Source: CAD feature listing. Evaluate the final solid. Frame: model axes, mm. Face numbers are marked on the shaded views. A direction names the side the tool comes from. Coordinates: 2 decimals unless noted, no trailing zeros. Order: outer loops, then holes, each group sorted by start corner. A loop starts at its lowest first (then second) coordinate and runs counter-clockwise, first axis right, second up.
```python
from build123d import *

# Parameters (mm, degrees)
BASE_FLANGE1_DEPTH           = 3.175
SKETCH7_R                    = 3.15
CUT_EXTRUDE3_DEPTH           = 10
EDGE_FLANGE1_STRIP_W         = 19.05
EDGE_FLANGE1_STRIP_H         = 3.175
EDGE_FLANGE1_STRIP_CUT_DEPTH = 36.40397533
EDGE_FLANGE1_DEPTH           = 36.40397533
SKETCH12_R                   = 2.65
CUT_EXTRUDE4_DEPTH           = 10


# Sheet-metal steps are written as plain solids
with BuildPart() as part:
    # Sketch2 → Base-Flange1 (new body)
    with BuildSketch(Plane(origin=(0, 0, 0), x_dir=(0, 0, -1), z_dir=(1, 0, 0))):
        with BuildLine():
            Line((0, 0), (0, 36.40397533))
            Line((0, 36.40397533), (49.693245392, 36.40397533))
            Line((49.693245392, 36.40397533), (24.989293369, 2.07924376))
            ThreePointArc((24.989293369, 2.07924376), (23.211005522, 0.550068473), (20.931069251, 0))
            Line((20.931069251, 0), (0, 0))
        make_face()
    extrude(amount=-BASE_FLANGE1_DEPTH)

    # Sketch7 → Cut-Extrude3 (cut)
    with BuildSketch(Plane.ZY.offset(3.175)):
        with Locations((-27.553898694, 30)):
            Circle(SKETCH7_R)
        with Locations((-12.587671369, 10)):
            Circle(SKETCH7_R)
    extrude(amount=-CUT_EXTRUDE3_DEPTH, mode=Mode.SUBTRACT)

    # Edge-Flange1 strip (across the edge) → Edge-Flange1 strip cut (cut)
    with BuildSketch(Plane(origin=(0, 36.40397533, 0), x_dir=(0, 0, -1), z_dir=(0, -1, 0))):
        with Locations((-3.175, -1.5875)):
            Rectangle(EDGE_FLANGE1_STRIP_W, EDGE_FLANGE1_STRIP_H)
    extrude(amount=EDGE_FLANGE1_STRIP_CUT_DEPTH, mode=Mode.SUBTRACT)

    # Edge-Flange1 section (across the edge) → Edge-Flange1 (add)
    with BuildSketch(Plane(origin=(0, 36.40397533, 0), x_dir=(0, 0, -1), z_dir=(0, -1, 0))):
        with BuildLine():
            Line((0, 3.175), (0, 15))
            Line((0, 15), (3.175, 15))
            Line((3.175, 15), (3.175, 3.175))
            ThreePointArc((3.175, 3.175), (4.10493597, 0.92993597), (6.35, 0))
            Line((6.35, 0), (6.35, -3.175))
            ThreePointArc((6.35, -3.175), (1.859871939, -1.315128061), (0, 3.175))
        make_face()
    extrude(amount=EDGE_FLANGE1_DEPTH)

    # Sketch12 → Cut-Extrude4 (cut)
    with BuildSketch(Plane(origin=(0, 0, -3.175), x_dir=(-1, 0, 0), z_dir=(0, 0, -1))):
        with Locations((-9.0875, 17.162271256)):
            Circle(SKETCH12_R)
    extrude(amount=-CUT_EXTRUDE4_DEPTH, mode=Mode.SUBTRACT)


solid = part.part
```
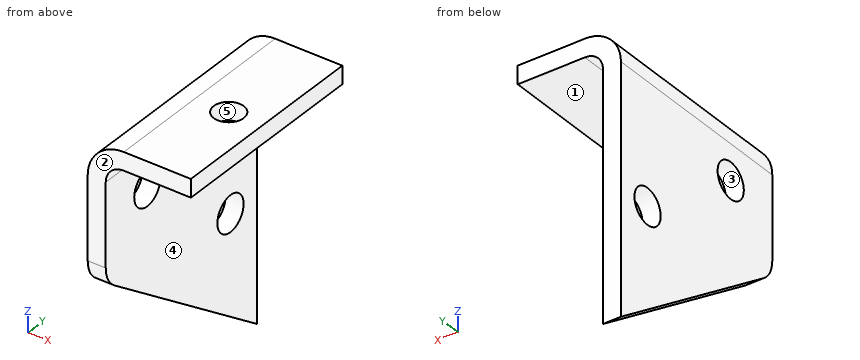
Q1. Section query D-D on y = 5. Output: boundary loops of the cut face in (x, z) (3 decimals).
Solutions:
outline: (-3.175, -27.091) - (0, -27.091) - (0, -6.35) arc R3.175 cw to (3.175, -3.175) - (15, -3.175) - (15, 0) - (3.175, 0) arc R6.35 ccw to (-3.175, -6.35) - close
Q2. Material intervals for line 1 along Z through (x, y) = (4.5, 32.5) (3 decimals); line 2 along Z through (x, y) = (-1.25, 20.5), sorted ascending.
Solutions:
line 1: z = -3.175 to 0
line 2: z = -38.25 to -1.8
Q3. Pin query (flat end, axial travel): P1, Ø1.5, axis at x = 2, y = 18, coming from the +Z side; P2, Ø11, axis at y = 14, z = -20.5, coming from the +X side; P3, Ø5, axis at y = 30, z = -27.55, coming from the +X side; P4, Ø7, axis at x = 9.09, y = 17.16, coming from the -Z side (3 decimals). Return the tip coordinate at first contact, or that it passes through.
Solutions:
P1: stops at z = -0.01
P2: stops at x = 0
P3: passes through
P4: stops at z = -3.175
Q4. Section query B-B on y = 11. Output: boundary loops of the cut face in (x, z) (3 decimals).
Solutions:
outline: (-3.175, -31.41) - (0, -31.41) - (0, -15.575) - (-3.175, -15.575) - close; (-3.175, -9.601) - (0, -9.601) - (0, -6.35) arc R3.175 cw to (3.175, -3.175) - (15, -3.175) - (15, 0) - (3.175, 0) arc R6.35 ccw to (-3.175, -6.35) - close
Q5. Section query C-C on z = -13. Output: boundary loops of the cut face in (x, y) (3 decimals).
Solutions:
outline: (-3.175, 0) - (0, 0) - (0, 6.877) - (-3.175, 6.877) - close; (-3.175, 13.123) - (0, 13.123) - (0, 36.404) - (-3.175, 36.404) - close
Q6. Set-up query: the marked faces 4 and 5. Return all of +Z, -Z, +X, -X, +Y, -Y with unobstructed straight access to the full face (end or side cutting, diameter ignored); none if empty.
Solutions:
face 4: -Z, +X, +Y, -Y
face 5: +Z, -Z
Q7. Pull-direction query (Z, two-part tool) for the marked faces 1, 2 and 3; classes: pulls with the +Z half, pulls with the -Z half, needs draft (parallel to the pull), parting line crosses it, or undercut.
Solutions:
face 1: pulls with the -Z half
face 2: needs draft
face 3: undercut
Q8. Section query A-A on x = 8. Output: boundary loops of the cut face in (y, z) (3 decimals), plus the area to 3 significant figures.
Solutions:
outline: (0, -3.175) - (14.746, -3.175) - (14.746, 0) - (0, 0) - close; (19.579, -3.175) - (36.404, -3.175) - (36.404, 0) - (19.579, 0) - close
area: 100 mm2
